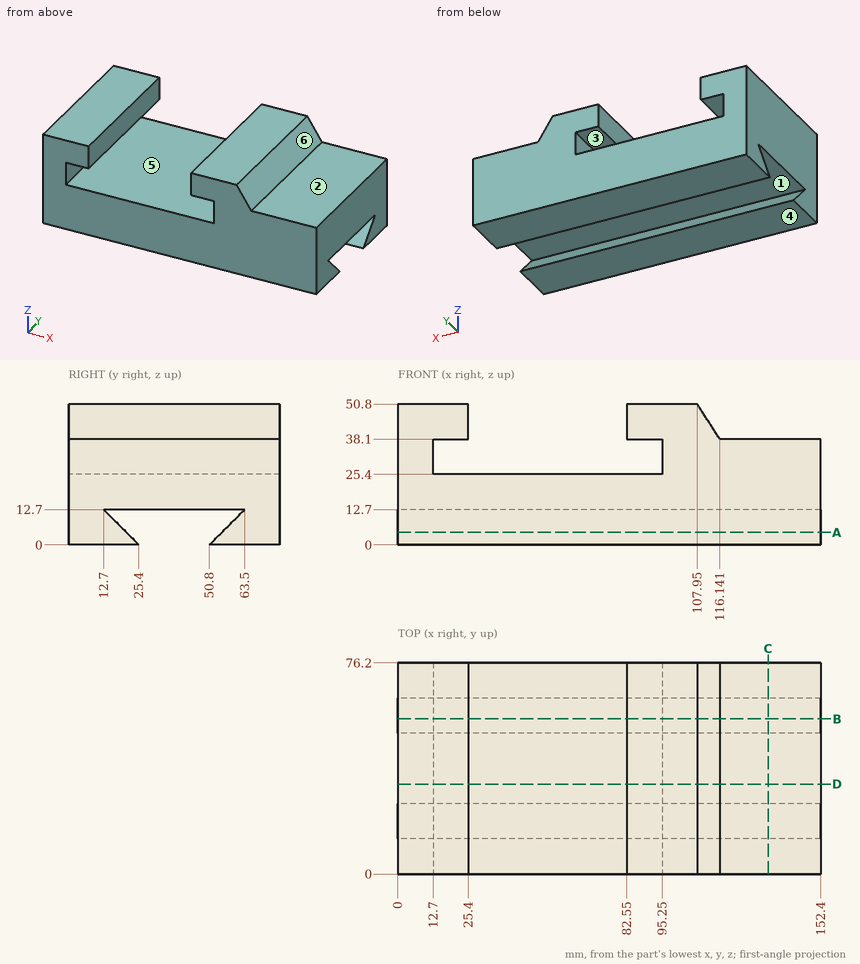
Print and shaded views of the part. All mm, measured from the part's lowest x, y and z. A direction names the side the tool comes from. Coordinates: 2 decimals unless noted, no trailing zeros. Loops run counter-clockwise (first coordinate to the right, second up) from the corner with the lowest first, then second, coordinate; pieces in that order, holes last. Notation, with made-up numbers: (60.5, -30) - (117.5, -30) arc R19 cw to (117.5, -3) - close; hole circle Ø6 at (71.25, 35.25). An arc over 180 degrees is marked (long way). Write item = value, one per line. Start each with the question number.
Item 1: Cut at C-C, the plane x = 133.5. Give the cut face in (y, z), and give its area (3 significant figures).
Item 2: 3-axis set-ups, long thin cutter, end or side, ignore diameter. For the marked faces 1, 2 and 3: which of +Z, -Z, +X, -X, +Y, -Y reach the whole face in a straight line?
Item 3: Cut at B-B, the plane y = 56. Give the cut face in (x, z), and give its area (3 significant figures).
Item 4: Cut at A-A, the plane z = 4.5. Give the cut face in (x, y).
Item 5: Cut at D-D, the plane y = 32.5. Give the cut face in (x, z), and give its area (3 significant figures).
Item 6: Wall check: L1, parallel to X at y = 26, z = 31.5; L2, parallel to Z at x = 85, y = 24; L3, parallel to Z at x = 13, y = 45. Give the ranges that are in metal, low to high. Write a range as from..to.
Item 7: Mould opens along X. For the marked faces 4, 5 and 6 say: released by +X, released by -X, zero draft, split by the parting line, or undercut.
Item 8: Flat gauge pins, fed straight in: pin 1 Ø1 at (x, y) = (116, 47) entering from +Z (1 decimal); pin 2 Ø6.5 at (y, z) = (56, 45.5) entering from -X; pin 3 Ø6.5 at (x, y) = (91.5, 38.5) entering from -Z; pin 4 Ø6.5 at (y, z) = (37.5, 44.5) entering from +X. Where does each tip first touch, or does it go through?
The answers:
q1.outline = (0, 0) - (25.4, 0) - (12.7, 12.7) - (63.5, 12.7) - (50.8, 0) - (76.2, 0) - (76.2, 38.1) - (0, 38.1) - close
q1.area = 2,420 mm2
q2.face_1 = +X, -X
q2.face_2 = +Z, +X, +Y, -Y
q2.face_3 = +Y, -Y
q3.outline = (0, 0) - (152.4, 0) - (152.4, 5.2) - (0, 5.2) - close; (0, 12.7) - (152.4, 12.7) - (152.4, 38.1) - (116.14, 38.1) - (107.95, 50.8) - (82.55, 50.8) - (82.55, 38.1) - (95.25, 38.1) - (95.25, 25.4) - (12.7, 25.4) - (12.7, 38.1) - (25.4, 38.1) - (25.4, 50.8) - (0, 50.8) - close
q3.area = 4,310 mm2
q4.outline = (0, 0) - (152.4, 0) - (152.4, 20.9) - (0, 20.9) - close; (0, 55.3) - (152.4, 55.3) - (152.4, 76.2) - (0, 76.2) - close
q5.outline = (0, 12.7) - (152.4, 12.7) - (152.4, 38.1) - (116.14, 38.1) - (107.95, 50.8) - (82.55, 50.8) - (82.55, 38.1) - (95.25, 38.1) - (95.25, 25.4) - (12.7, 25.4) - (12.7, 38.1) - (25.4, 38.1) - (25.4, 50.8) - (0, 50.8) - close
q5.area = 3,520 mm2
q6.L1 = 0..12.7, 95.25..152.4
q6.L2 = 0..1.4, 12.7..25.4, 38.1..50.8
q6.L3 = 12.7..25.4, 38.1..50.8
q7.face_4 = zero draft
q7.face_5 = undercut
q7.face_6 = released by +X
q8.pin_1 = 39.1
q8.pin_2 = 0
q8.pin_3 = 12.7
q8.pin_4 = 114.11
